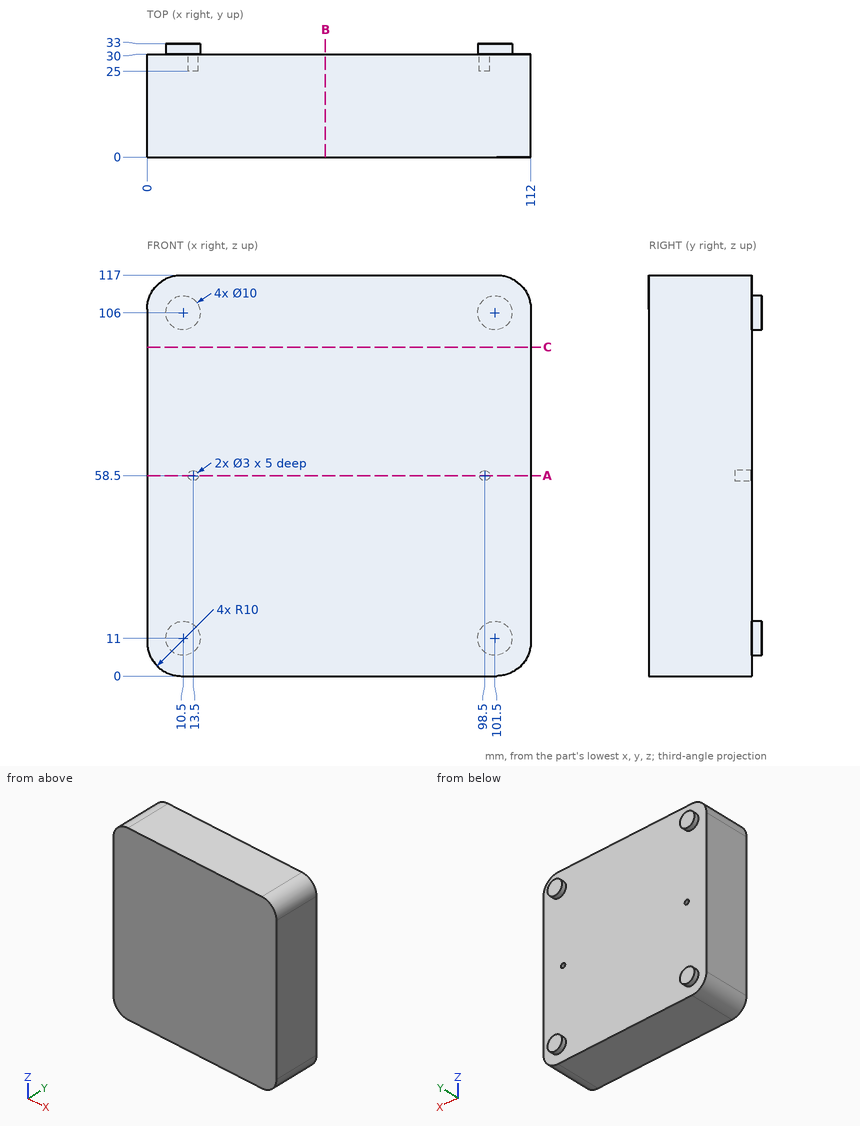
Design review of the part shown in the three views and the two pictorial views. Dimensions are in mm from the part's minimum x, y and z. Give positions to 0.01 mm unless a question says otherwise; leave off trailing zeros. Loops run counter-clockwise (first coordinate to the right, second up) from the corner with the lowest first, then second, coordinate; pieces in that order, holes last. Notation, with made-up numbers: (18.5, 6.25) -> (68.5, 6.25) arc R21 ccw to (68.5, 12.25) -> close; hole circle Ø9 at (14.25, 4). An arc over 180 degrees is marked (long way). Put each result on its own line as item: value. Start each with the question number.
1. We need section B-B on x = 52. State the section outline as (y, z) points, then the cut area to 3 significant figures.
2. Clearance check with a flat-ended pin moving along its axis: P1, Ø0.9, axis at x = 13.5, z = 59, coming from the +Y side. State where the tip first meets the part, or that it passes through.
3. We need section C-C on z = 96. State the section outline as (x, y) points, then the cut area to 3 significant figures.
4. Wall thickness on probe 1 along X at (y, z) = (28.25, 58.5); probe 2 along Y at (x, z) = (43, 82); probe 3 along Z at (x, y) = (98.5, 27.35): over which ranges is each line inside the solid? List them lowest first.
5. We need section A-A on z = 58.5. State the section outline as (x, y) points, then the cut area to 3 significant figures.
Determined:
1. outline: (0, 0) -> (30, 0) -> (30, 117) -> (0, 117) -> close
1. area: 3,510 mm^2
2. P1: y = 25
3. outline: (0, 0) -> (112, 0) -> (112, 30) -> (0, 30) -> close
3. area: 3,360 mm^2
4. probe 1: 0 to 12, 15 to 97, 100 to 112
4. probe 2: 0 to 30
4. probe 3: 0 to 57, 60 to 117
5. outline: (0, 0) -> (112, 0) -> (112, 30) -> (100, 30) -> (100, 25) -> (97, 25) -> (97, 30) -> (15, 30) -> (15, 25) -> (12, 25) -> (12, 30) -> (0, 30) -> close
5. area: 3,330 mm^2
